from build123d import *

# Parameters (mm, degrees)
SKETCH1_W           = 9.8
SKETCH1_H           = 11.8
BOSS_EXTRUDE1_DEPTH = 0.5
SKETCH2_R           = 1.5
BOSS_EXTRUDE2_DEPTH = 55
SKETCH5_R           = 0.5
CUT_EXTRUDE1_DEPTH  = 55
SKETCH6_R           = 1.5
BOSS_EXTRUDE3_DEPTH = 7
BOSS_EXTRUDE4_DEPTH = 16


with BuildPart() as part:
    # Sketch1 → Boss-Extrude1 (new body)
    with BuildSketch(Plane(origin=(0, 0, 0), x_dir=(1, 0, 0), z_dir=(0, 1, 0))):
        Rectangle(SKETCH1_W, SKETCH1_H)
    extrude(amount=BOSS_EXTRUDE1_DEPTH)

    # Sketch2 → Boss-Extrude2 (add)
    with BuildSketch(Plane.XZ):
        Circle(SKETCH2_R)
    extrude(amount=BOSS_EXTRUDE2_DEPTH)

    # Sketch5 → Cut-Extrude1 (cut)
    with BuildSketch(Plane.XZ):
        with Locations((0, 4.4)):
            Circle(SKETCH5_R)
        with Locations((0, -4.4)):
            Circle(SKETCH5_R)
    extrude(amount=-CUT_EXTRUDE1_DEPTH, mode=Mode.SUBTRACT)

    # Sketch6 → Boss-Extrude3 (add)
    with BuildSketch(Plane(origin=(0, 0.5, 0), x_dir=(1, 0, 0), z_dir=(0, 1, 0))):
        with Locations((-2.983296991, -3.592133112)):
            Circle(SKETCH6_R)
        with Locations((2.983296991, 3.592133112)):
            Circle(SKETCH6_R)
    extrude(amount=BOSS_EXTRUDE3_DEPTH)

    # Sketch7 → Boss-Extrude4 (add)
    with BuildSketch(Plane(origin=(0, 7.5, 0), x_dir=(1, 0, 0), z_dir=(0, 1, 0))):
        with BuildLine():
            Line((-1.9, 5.9), (1.9, 5.9))
            ThreePointArc((1.9, 5.9), (4.021320344, 5.021320344), (4.9, 2.9))
            Line((4.9, 2.9), (4.9, -2.907128276))
            ThreePointArc((4.9, -2.907128276), (4.021320344, -5.028448619), (1.9, -5.907128276))
            Line((1.9, -5.907128276), (-1.9, -5.907128276))
            ThreePointArc((-1.9, -5.907128276), (-4.021320344, -5.028448619), (-4.9, -2.907128276))
            Line((-4.9, -2.907128276), (-4.9, 2.9))
            ThreePointArc((-4.9, 2.9), (-4.021320344, 5.021320344), (-1.9, 5.9))
        make_face()
    extrude(amount=BOSS_EXTRUDE4_DEPTH)


solid = part.part
Can you work these out from the model? Positions are in its coordinate system, mm. A direction names the side the tool comes from. Give positions to 0.01 mm unless a question says otherwise; leave off trailing zeros. Loops run counter-clockwise (first coordinate to the right, second up) from the corner with the lowest first, then second, coordinate; pieces in that order, holes last. Notation, with made-up numbers: (-28, 84.25) - (-11, 84.25) arc R28 ccw to (-11, 113.25) - close; hole circle Ø9 at (57, -8). An arc over 180 degrees is marked (long way). Answer as a JSON object with one key per item and string values.
Q1. If we mould it in two halves opening along Y, with no side actions, what happens to faces 6 (the cylindrical face through (-4.482, 3.951, 3.526)), 7 (the cylindrical face through (4.045, 15.388, 5.005)), 8 (the cylindrical face through (1.79, 3.95, -2.68)), 9 (the flat face through (0, -55, 0))? For each: pulls with the +Y half, pulls with the -Y half, needs draft (parallel to the pull), parting line crosses it, or undercut.
Geometry says:
{"face 6": "undercut", "face 7": "needs draft", "face 8": "undercut", "face 9": "pulls with the -Y half"}
Q2. Imagine slicing it at C-C on x = -2.75. Write out the boundary of the cut face in (y, z), plus the area to 3 significant figures.
Geometry says:
{"outline": "(0, -5.9) - (0.5, -5.9) - (0.5, 2.11) - (7.5, 2.11) - (7.5, -5.78) - (23.5, -5.78) - (23.5, 5.78) - (7.5, 5.78) - (7.5, 5.07) - (0.5, 5.07) - (0.5, 5.9) - (0, 5.9) - close", "area": "212 mm²"}
Q3. If I drill on L1, parallel to Z at x = 0, y = 0.35; L2, parallel to Y at x = 4.25, z = 4.25; L3, parallel to Y at x = -2.25, z = 3.25, over which ranges is the centre line in solid material (lowest first)?
Geometry says:
{"L1": "-5.9 to -4.9, -3.9 to 3.9, 4.9 to 5.9", "L2": "0 to 0.5, 7.5 to 23.5", "L3": "0 to 23.5"}
Q4. Will these pins go through, and if not, where does the flat tip stop? P1, Ø2, axis at x = 3, y = -44, coming from the -Z side; P2, Ø3, axis at x = 2, z = -3, coming from the -Y side; P3, Ø6, axis at y = -38, z = 1, coming from the +X side.
Geometry says:
{"P1": "through", "P2": "y = 0", "P3": "x = 1.5"}
Q5. Which directions (+Z, -Z, +X, -X, +Y, -Y) give clear straight access to the entire face, cutting with the end or side of a thin tool? Please do faces 1 (the cylindrical face through (4, 15.39, -5.04)), 2 (the cylindrical face through (-4, 15.39, 5.05)), 3 (the flat face through (-1.2, 0, 1.2)), 4 (the cylindrical face through (-4.04, 15.39, -5)), 5 (the flat face through (0, 0.5, 0)).
Geometry says:
{"face 1": "-Z, +X, +Y", "face 2": "+Z, -X, +Y", "face 3": "-Y", "face 4": "-Z, -X, +Y", "face 5": "none"}
Q6. Imagine slicing it at A-A on z = 0. Write out the boundary of the cut face in (x, y).
Geometry says:
{"outline": "(-4.9, 0) - (-1.5, 0) - (-1.5, -55) - (1.5, -55) - (1.5, 0) - (4.9, 0) - (4.9, 0.5) - (-4.9, 0.5) - close; (-4.9, 7.5) - (4.9, 7.5) - (4.9, 23.5) - (-4.9, 23.5) - close"}
Q7. Imagine slicing it at B-B on y = 13. Write out the boundary of the cut face in (x, z).
Geometry says:
{"outline": "(-4.9, -2.9) arc R3 ccw to (-1.9, -5.9) - (1.9, -5.9) arc R3 ccw to (4.9, -2.9) - (4.9, 2.91) arc R3 ccw to (1.9, 5.91) - (-1.9, 5.91) arc R3 ccw to (-4.9, 2.91) - close"}
Q8. Imagine slicing it at D-D on y = -38. Write out the boundary of the cut face in (x, z).
Geometry says:
{"outline": "circle Ø3 at (0, 0)"}
